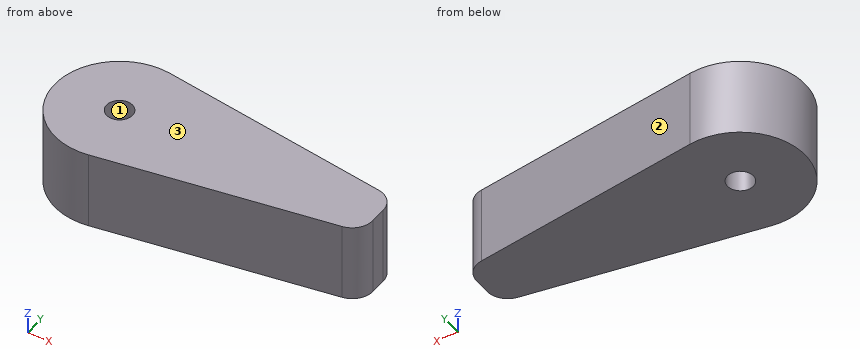
Autodesk Inventor part; units mm, degrees
ref_plane "YZ Plane" through (0, 0, 0) normal (1, 0, 0) x (0, 1, 0)
ref_plane "XZ Plane" through (0, 0, 0) normal (0, 1, 0) x (-1, 0, 0)
ref_plane "XY Plane" through (0, 0, 0) normal (0, 0, 1) x (1, 0, 0)
sketch "Sketch1" plane through (0, 0, 0) normal (0, 0, 1) x (1, 0, 0)
  circle A0 centre (0, 0) radius 12.5
  line L0 (0, 0) -> (50, 0) construction
  line L1 (1.8894, 12.3564) -> (50, 5)
  line L2 (1.8894, -12.3564) -> (50, -5)
  line L3 (50, 5) -> (50, -5)
  dimension "d0" = 25
  dimension "d1" = 50
  dimension "d2" = 5
  dimension "d3" = 5
  dimension "d4" = 50
extrude "Extrusion1" add sketch "Sketch1" along normal blind 15
fillet "Fillet1" radius 4 2 edges at (50, 5, 7.5) (50, -5, 7.5)
sketch "Sketch2" plane through (0, 0, 15) normal (0, 0, 1) x (1, 0, 0)
  circle A0 centre (0, 0) radius 2.5
  dimension "d8" = 5
extrude "Extrusion2" cut sketch "Sketch2" against normal through all
properties part number "o_Plattenstopper" material "Birch"
Source: CAD feature listing. Evaluate the final solid. Frame: model axes, mm. Face numbers are marked on the shaded views. Give positions to 0.01 mm unless a question says otherwise; leave off trailing zeros. Write each loop counter-clockwise with the first axis right and the second up, starting at its lowest first coordinate (ties: lowest second). Pieces come first, ordered by that corner, then holes. Notation, with made-up numbers: (79, 52.5) - (108, 52.5) arc R21 cw to (108, 81.5) - close; hole circle Ø5 at (89, 73). An arc over 180 degrees is marked (long way). Write item = value, one per line. Start each with the question number.
Q1. Cut plane C-C, the plane z = 2.75. Return loops of the section in (x, y), then the cut area to 3 significant figures.
Q2. Cut plane A-A, the plane x = 0. Return loops of the section in (y, z).
Q3. Cut plane D-D, the plane y = 9.25. Return loops of the section in (x, z).
Q4. Pin query (flat end, axial travel): pin 1 Ø4 at (x, z) = (15, 6) entering from +Y; pin 2 Ø1.5 at (x, z) = (18, 2.5) entering from -Y. Return the tip coordinate at first contact, or that it passes through.
Q5. Material intervals for probe 1 along Y at (x, z) = (0, 7); probe 2 along X at (y, z) = (0.25, 13.5); probe 3 along Y at (x, z) = (23.5, 10.25), sorted ascending.
Q6. Draft query along X for the marked faces 1, 2 and 3. Return one class per face: +X half, -X half, draft (parallel to the pull), parting line (faces both ways), or undercut.
Q7. Cut plane B-B, the plane y = 0. Return loops of the section in (x, z).
Computed values:
q1.outline = (1.89, -12.36) - (46.6, -5.52) arc R4 ccw to (50, -1.57) - (50, 1.57) arc R4 ccw to (46.6, 5.52) - (1.89, 12.36) arc R12.5 ccw (long way) to start; hole circle Ø5 at (0, 0)
q1.area = 1,100 mm²
q2.outline = (-12.5, 0) - (-2.5, 0) - (-2.5, 15) - (-12.5, 15) - close; (2.5, 0) - (12.5, 0) - (12.5, 15) - (2.5, 15) - close
q3.outline = (-8.41, 0) - (22.21, 0) - (22.21, 15) - (-8.41, 15) - close
q4.pin_1 = 10.66
q4.pin_2 = -10.01
q5.probe_1 = -12.5 to -2.5, 2.5 to 12.5
q5.probe_2 = -12.5 to -2.49, 2.49 to 50
q5.probe_3 = -9.05 to 9.05
q6.face_1 = undercut
q6.face_2 = +X half
q6.face_3 = draft
q7.outline = (-12.5, 0) - (-2.5, 0) - (-2.5, 15) - (-12.5, 15) - close; (2.5, 0) - (50, 0) - (50, 15) - (2.5, 15) - close
